Geometry check sheet. Reference: the model listing, model coordinates, mm. Face numbers are marked on the shaded views. A direction names the side the tool comes from. Give positions to 0.01 mm unless a question says otherwise; leave off trailing zeros. Loops run counter-clockwise (first coordinate to the right, second up) from the corner with the lowest first, then second, coordinate; pieces in that order, holes last. Notation, with made-up numbers: (53.25, -20.75) -> (71.25, -20.75) arc R19 cw to (71.25, -16.75) -> close; hole circle Ø9 at (-25.75, 46.5). An arc over 180 degrees is marked (long way). Write each question's results on one line, items separated by ' | '. Start each with the question number.
1) Sectioned sample at C-C on z = 2.75. Count the separate pieces of the cut face and the enclosed holes in it, then the cut area to 3 significant figures.
2) Scan lines: line 1 (Y direction, x = 64.8, z = 3); line 2 (Y direction, x = 20, z = 0.75); line 3 (Y direction, x = 63.5, z = 7.75). Record each from-to range of solid material in increasing order. Write a range as from..to.
3) Sectioned sample at B-B on y = -0.95. Record the cut outline in (x, z), then the cut area to 3 significant figures.
4) Sectioned sample at D-D on x = 64.8. Record the cut outline in (y, z), then the cut area to 3 significant figures.
5) Depth check by flat-ended pin: pin 1 (7 mm diameter, centred on x = -20, y = -0.95, fed in from +Z); pin 2 (13 mm diameter, centred on x = 44.5, y = 4.5, fed in from -Z). Enter the tip coordinate at first touch or a pass-through.
6) Set-up check for the marked faces 1, 2 and 3: record each of +Z, -Z, +X, -X, +Y, -Y from which the full face is reachable in a straight line by a thin tool's end or side.
7) Sectioned sample at A-A on x = -20. Record the cut outline in (y, z), then the cut area to 3 significant figures.
```python
from build123d import *

# Parameters (mm, degrees)
SKETCH1_W           = 147.6
SKETCH1_H           = 78.1
BOSS_EXTRUDE1_DEPTH = 12
SKETCH2_W           = 60
SKETCH2_H           = 78.1
BOSS_EXTRUDE2_DEPTH = 5
SKETCH3_R           = 2.5
CUT_EXTRUDE1_DEPTH  = 86.207643436
SKETCH4_R           = 4
CUT_EXTRUDE2_DEPTH  = 86.207643436
SKETCH5_R           = 5.9
CUT_EXTRUDE3_DEPTH  = 5


with BuildPart() as part:
    # Sketch1 → Boss-Extrude1 (new body)
    with BuildSketch(Plane.XY):
        Rectangle(SKETCH1_W, SKETCH1_H)
    extrude(amount=BOSS_EXTRUDE1_DEPTH)

    # Sketch2 → Boss-Extrude2 (add)
    with BuildSketch(Plane(origin=(0, 0, 0), x_dir=(-1, 0, 0), z_dir=(0, 0, -1))):
        Rectangle(SKETCH2_W, SKETCH2_H)
    extrude(amount=BOSS_EXTRUDE2_DEPTH)

    # Sketch3 → Cut-Extrude1 (cut, through all)
    with BuildSketch(Plane(origin=(0, 0, -5), x_dir=(-1, 0, 0), z_dir=(0, 0, -1))):
        with Locations((-20, 19.05)):
            Circle(SKETCH3_R)
        with Locations((-20, -0.95)):
            Circle(SKETCH3_R)
        with Locations((-20, -20.95)):
            Circle(SKETCH3_R)
        with Locations(Location((20, -20.95, 0), (0, 0, 180))):
            Circle(SKETCH3_R)
        with Locations(Location((20, -0.95, 0), (0, 0, 180))):
            Circle(SKETCH3_R)
        with Locations(Location((20, 19.05, 0), (0, 0, 180))):
            Circle(SKETCH3_R)
    extrude(amount=-CUT_EXTRUDE1_DEPTH, mode=Mode.SUBTRACT)

    # Sketch4 → Cut-Extrude2 (cut, through all)
    with BuildSketch(Plane.XY.offset(12)):
        with Locations((64.8, 24.05)):
            Circle(SKETCH4_R)
        with Locations((64.8, -25.95)):
            Circle(SKETCH4_R)
        with Locations(Location((-64.8, -25.95, 0), (0, 0, 180))):
            Circle(SKETCH4_R)
        with Locations(Location((-64.8, 24.05, 0), (0, 0, 180))):
            Circle(SKETCH4_R)
    extrude(amount=-CUT_EXTRUDE2_DEPTH, mode=Mode.SUBTRACT)

    # Sketch5 → Cut-Extrude3 (cut)
    with BuildSketch(Plane.XY.offset(12)):
        with Locations((-20, 19.05)):
            Circle(SKETCH5_R)
        with Locations((20, 19.05)):
            Circle(SKETCH5_R)
        with Locations((-20, -0.95)):
            Circle(SKETCH5_R)
        with Locations((20, -0.95)):
            Circle(SKETCH5_R)
        with Locations((-20, -20.95)):
            Circle(SKETCH5_R)
        with Locations((20, -20.95)):
            Circle(SKETCH5_R)
    extrude(amount=-CUT_EXTRUDE3_DEPTH, mode=Mode.SUBTRACT)


solid = part.part
```
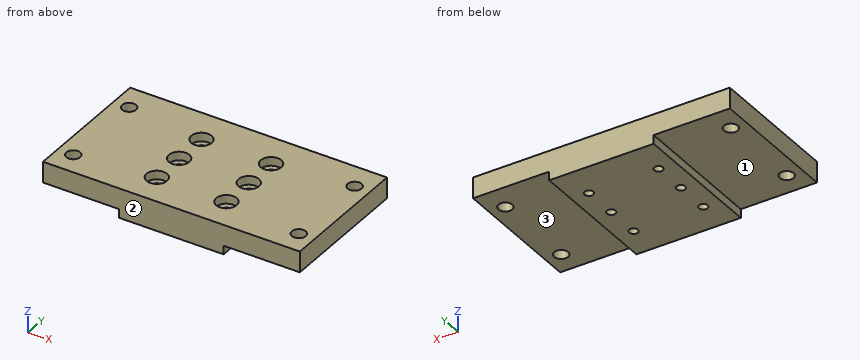
Result:
1) separate pieces: 1 | enclosed holes: 10 | area: 11,200 mm^2
2) line 1: -39.05..-29.95, -21.95..20.05, 28.05..39.05 | line 2: -39.05..-23.45, -18.45..-3.45, 1.55..16.55, 21.55..39.05 | line 3: -39.05..-29.73, -22.17..20.27, 27.83..39.05
3) outline: (-73.8, 0) -> (-30, 0) -> (-30, -5) -> (-22.5, -5) -> (-22.5, 7) -> (-25.9, 7) -> (-25.9, 12) -> (-73.8, 12) -> close; (-17.5, -5) -> (17.5, -5) -> (17.5, 7) -> (14.1, 7) -> (14.1, 12) -> (-14.1, 12) -> (-14.1, 7) -> (-17.5, 7) -> close; (22.5, -5) -> (30, -5) -> (30, 0) -> (73.8, 0) -> (73.8, 12) -> (25.9, 12) -> (25.9, 7) -> (22.5, 7) -> close | area: 1,830 mm^2
4) outline: (-39.05, 0) -> (-29.95, 0) -> (-29.95, 12) -> (-39.05, 12) -> close; (-21.95, 0) -> (20.05, 0) -> (20.05, 12) -> (-21.95, 12) -> close; (28.05, 0) -> (39.05, 0) -> (39.05, 12) -> (28.05, 12) -> close | area: 745 mm^2
5) pin 1: z = 7 | pin 2: z = 0
6) face 1: -Z, -X, +Y, -Y | face 2: +Z, -Z, +X, -X, -Y | face 3: -Z, +X, +Y, -Y
7) outline: (-39.05, -5) -> (-23.45, -5) -> (-23.45, 7) -> (-26.85, 7) -> (-26.85, 12) -> (-39.05, 12) -> close; (-18.45, -5) -> (-3.45, -5) -> (-3.45, 7) -> (-6.85, 7) -> (-6.85, 12) -> (-15.05, 12) -> (-15.05, 7) -> (-18.45, 7) -> close; (1.55, -5) -> (16.55, -5) -> (16.55, 7) -> (13.15, 7) -> (13.15, 12) -> (4.95, 12) -> (4.95, 7) -> (1.55, 7) -> close; (21.55, -5) -> (39.05, -5) -> (39.05, 12) -> (24.95, 12) -> (24.95, 7) -> (21.55, 7) -> close | area: 971 mm^2
